Input: part model. Units: mm. Frame: model coordinates. A direction names the side the tool comes from. Coordinates: 2 decimals unless noted, no trailing zeros. Write each loop counter-clockwise with the first axis right and the second up, starting at its lowest first coordinate (ties: lowest second). Pieces come first, ordered by that corner, then holes. Notation, with made-up numbers: (17, 47.5) - (21, 47.5) arc R20 ccw to (21, 59.5) - close; hole circle Ø9 at (33, -3.5). An arc over 180 degrees is marked (long way). Put each result on its own line as item: value. Start each with the question number.
1. Access query for faces 1 (the cylindrical face through (60.42, -0.27, 7.67)), 2 (the flat face through (47, 2.01, 9)), 3 (the flat face through (12, -2.49, 9)), 4 (the flat face through (13, 2.01, 9)), 5 (the flat face through (46, -2.49, 9)). Directions: +Z, -Z, +X, -X, +Y, -Y. A direction counts if a zero-diameter tool reaches every point of the face in a straight line with its end or side. Return the directions, or none.
2. Cut plane C-C, the plane z = 33.5. Return loops of the section in (x, y) (1 decimal), and give its area (3 significant figures).
3. Cut plane D-D, the plane x = -1. Return loops of the section in (y, z).
4. Pin query (flat end, axial travel): pin 1 (6 mm diameter, centred on x = 2.5, z = 7.5, fed in from +Y); pin 2 (5.5 mm diameter, centred on x = 12, z = 12, fed in from -Y); pin 3 (2 mm diameter, centred on y = 3, z = 54, fed in from +X). Return the tip coordinate at first contact, or that it passes through.
5. Cut plane A-A, the plane y = 1. Return loops of the section in (x, z).
6. Line query: line 1 (Y direction, x = 25, z = 12); line 2 (Z direction, x = 24, y = -2.25); line 3 (X direction, y = -0.5, z = 58). Output: solid intervals per line, ascending.
7. Cut plane B-B, the plane x = 38. Return loops of the section in (y, z), and give its area (3 significant figures).
from build123d import *

# Parameters (mm, degrees)
F1_DEPTH = 19
F2_R     = 4.7625
F3_DEPTH = 50
F5_DEPTH = 7.0135
F6_R     = 1.2


with BuildPart() as f1:
    # F0 (on Top) → F1 (new body)
    with BuildSketch(Plane.XY):
        with BuildLine():
            Line((25.3387194722, 2.0096014291), (-7.9637924397, 2.0096014291))
            Line((-7.9637924397, 2.0096014291), (-7.9637924397, -2.4903985709))
            Line((-7.9637924397, -2.4903985709), (25.3387194722, -2.4903985709))
            ThreePointArc((25.3387194722, -2.4903985709), (29.5362075603, -5.0028985709), (33.7336956484, -2.4903985709))
            Line((33.7336956484, -2.4903985709), (67.0362075603, -2.4903985709))
            Line((67.0362075603, -2.4903985709), (67.0362075603, 2.0096014291))
            Line((67.0362075603, 2.0096014291), (33.7336956484, 2.0096014291))
            ThreePointArc((33.7336956484, 2.0096014291), (29.5362075603, 4.5221014291), (25.3387194722, 2.0096014291))
        make_face()
    extrude(amount=F1_DEPTH)

    # F2 (on face) → F3 (join)
    with BuildSketch(Plane.XY.offset(19)):
        with Locations((29.5362075603, -0.2403985709)):
            Circle(F2_R)
    extrude(amount=F3_DEPTH)

    # F4 (on face) → F5 (cut, through all)
    with BuildSketch(Plane.XZ.offset(2.4903985709)):
        with BuildLine():
            ThreePointArc((68.2658283432, 20.1410173709), (61.3045105, 8.6713769002), (51.0663553295, 0))
            Line((51.0663553295, 0), (68.7501132488, 0))
            Line((68.7501132488, 0), (68.2658283432, 20.1410173709))
        make_face()
        with BuildLine():
            ThreePointArc((8.0060597912, 0), (-2.1784408901, 8.6086716648), (-9.1312425211, 19.9881194299))
            Line((-9.1312425211, 19.9881194299), (-9.1312425211, 0))
            Line((-9.1312425211, 0), (8.0060597912, 0))
        make_face()
    extrude(amount=-F5_DEPTH, mode=Mode.SUBTRACT)

    # F6
    f6_edges = [f1.edges().sort_by_distance(p)[0] for p in [
        (67.036208, -0.240399, 19),
        (-7.963792, -0.240399, 19),
    ]]
    fillet(f6_edges, radius=F6_R)


solid = f1.part
Report:
1. face 1: -Z, +X, +Y, -Y
1. face 2: +Z, -Z, +X, +Y
1. face 3: +Z, -Z, -X, -Y
1. face 4: +Z, -Z, -X, +Y
1. face 5: +Z, -Z, +X, -Y
2. outline: circle Ø9.5 at (29.5, -0.2)
2. area: 71.3 mm^2
3. outline: (-2.49, 7.29) - (2.01, 7.29) - (2.01, 19) - (-2.49, 19) - close
4. pin 1: stops at y = 2.01
4. pin 2: stops at y = -2.49
4. pin 3: stops at x = 33.74
5. outline: (-7.96, 17.39) arc R41.78 ccw to (8.01, 0) - (51.07, 0) arc R41.78 ccw to (67.04, 17.39) - (67.04, 17.8) arc R1.2 ccw to (65.84, 19) - (34.13, 19) - (34.13, 69) - (24.94, 69) - (24.94, 19) - (-6.76, 19) arc R1.2 ccw to (-7.96, 17.8) - close
6. line 1: y = -2.49 to 2.01
6. line 2: z = 0 to 19
6. line 3: x = 24.78 to 34.29
7. outline: (-2.49, 0) - (2.01, 0) - (2.01, 19) - (-2.49, 19) - close
7. area: 85.5 mm^2
